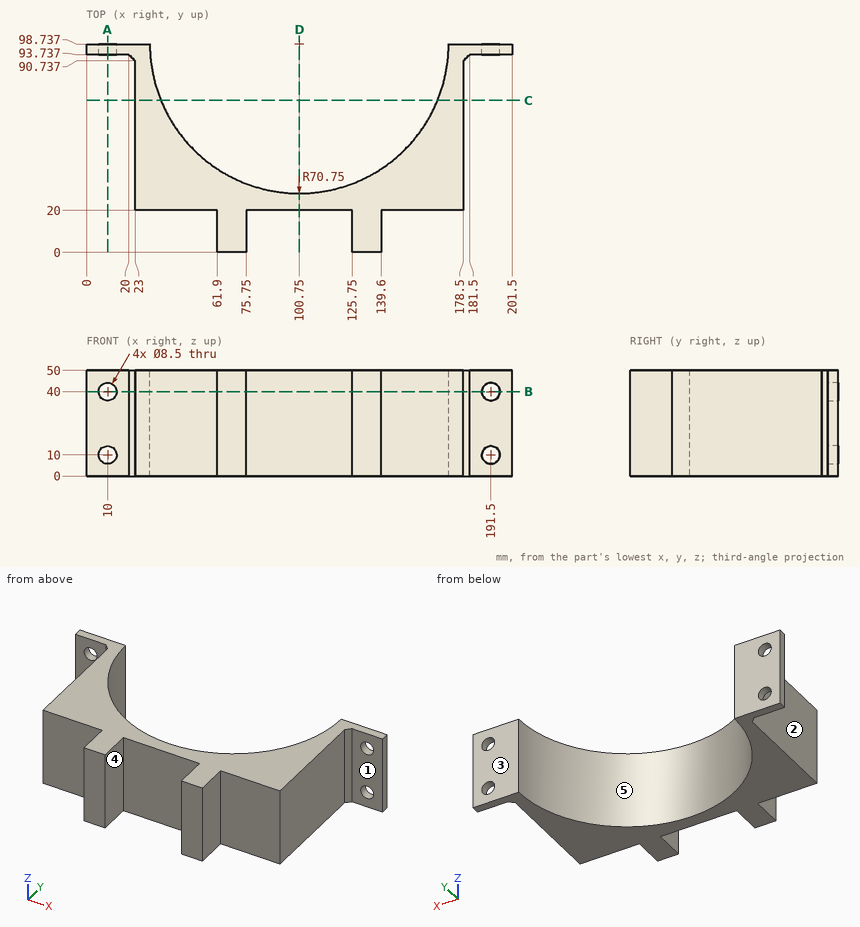
Answer from the drawing. Dimensions are ordinates in mm from the lowest x, y and z of the part. A direction names the side the tool comes from. Give positions to 0.01 mm unless a question says otherwise; leave off trailing zeros. Loops run counter-clockwise (first coordinate to the right, second up) from the corner with the lowest first, then second, coordinate; pieces in that order, holes last.
Item 1: For the marked faces 1, 2, 3, 4 and 5, determine the directions among +Z, -Z, +X, -X, +Y, -Y from which every point of the face is accessible in a straight line to the end or side of a thin tool.
Item 2: The part is cut by section B-B (z = 40). Write down the section's boundary in (x, y), and give its area (3 significant figures).
Item 3: Each of these flat-tipped pins is pushed along its axis until it touches: pin 1 Ø10 at (x, z) = (42.5, 27.5) entering from -Y; pin 2 Ø5 at (x, z) = (191.5, 40) entering from +Y; pin 3 Ø16 at (y, z) = (8.5, 14) entering from +X; pin 4 Ø12 at (x, y) = (103.5, 30) entering from +Z. Where does it stop, or does it pass through?
Item 4: Find the intervals of material crossed by line 1 along Z through (x, y) = (191, 95); line 2 along X through (y, z) = (97, 10); line 3 along X through (y, z) = (18, 16), in increasing order.
Item 5: The part is cut by section C-C (y = 72). Write down the section's boundary in (x, z), and give its area (3 significant figures).
Item 6: The part is cut by section A-A (x = 10). Write down the section's boundary in (y, z), and give its area (3 significant figures).
Item 7: The part is cut by section D-D (x = 100.75). Write down the section's boundary in (y, z).
Taken from the geometry:
1. face 1: +Z, -Z, +X, -Y
1. face 2: +Z, -Z, -X, -Y
1. face 3: +Z, -Z, +X, -X, +Y
1. face 4: +Z, -Z, -Y
1. face 5: +Z, -Z, +Y
2. outline: (0, 93.74) - (5.75, 93.74) - (5.75, 98.74) - (0, 98.74) - close; (14.25, 93.74) - (20, 93.74) - (23, 90.74) - (23, 20) - (61.9, 20) - (61.9, 0) - (75.75, 0) - (75.75, 20) - (125.75, 20) - (125.75, 0) - (139.6, 0) - (139.6, 20) - (178.5, 20) - (178.5, 90.74) - (181.5, 93.74) - (187.25, 93.74) - (187.25, 98.74) - (171.5, 98.74) arc R70.75 cw to (30, 98.74) - (14.25, 98.74) - close; (195.75, 93.74) - (201.5, 93.74) - (201.5, 98.74) - (195.75, 98.74) - close
2. area: 5,090 mm2
3. pin 1: stops at y = 20
3. pin 2: passes through
3. pin 3: stops at x = 139.6
3. pin 4: stops at z = 50
4. line 1: z = 0 to 5.78, 14.22 to 35.78, 44.22 to 50
4. line 2: x = 0 to 5.75, 14.25 to 30.02, 171.48 to 187.25, 195.75 to 201.5
4. line 3: x = 61.9 to 75.75, 125.75 to 139.6
5. outline: (23, 0) - (35.25, 0) - (35.25, 50) - (23, 50) - close; (166.25, 0) - (178.5, 0) - (178.5, 50) - (166.25, 50) - close
5. area: 1,220 mm2
6. outline: (93.74, 0) - (98.74, 0) - (98.74, 5.75) - (93.74, 5.75) - close; (93.74, 14.25) - (98.74, 14.25) - (98.74, 35.75) - (93.74, 35.75) - close; (93.74, 44.25) - (98.74, 44.25) - (98.74, 50) - (93.74, 50) - close
6. area: 165 mm2
7. outline: (20, 0) - (27.99, 0) - (27.99, 50) - (20, 50) - close
